Check sheet for the modelled part. Datum: model origin and axes. Units: mm. Round coordinates to 2 decimals unless told otherwise and drop trailing zeros. Write each loop counter-clockwise with the first axis right and the second up, starting at its lowest first coordinate (ties: lowest second). Pieces come first, ordered by that corner, then holes.
Item 1: Section check C-C, the plane y = -19.75. Record the cut outline in (x, z).
Item 2: Section check A-A, the plane z = -7. Record the cut outline in (x, y).
Item 3: Depth check by flat-ended pin: pin 1 (6.5 mm diameter, centred on y = -34.75, z = 83, fed in from -X); pin 2 (3 mm diameter, centred on x = 18.5, z = 81, fed in from +Y); pin 3 (3.5 mm diameter, centred on y = -34.75, z = 53, fed in from -X). Enter the tip coordinate at first touch or a pass-through.
Item 4: Section check B-B, the plane z = 68. Record the cut outline in (x, y), plus the area to 3 significant figures.
Item 5: Material ranges on line 1 along Y through (x, z) = (17.75, -7); line 2 along Z through (x, y) = (17, -19.75); line 3 along Y through (x, z) = (14.5, 83), recorded low to high.
Item 6: Section check D-D, the plane x = 16. State how many separate pieces and enclosed holes the cut face has, plus the area to 3 significant figures.
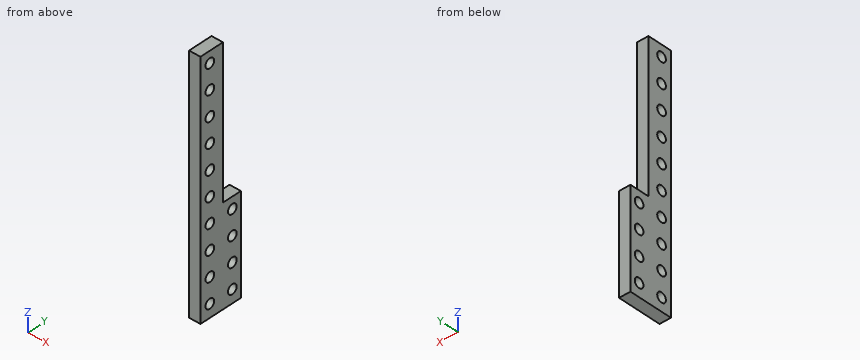
from build123d import *

# Parameters (mm, degrees)
CYLINDER021_R     = 2.9
CYLINDER021_DEPTH = 132
CYLINDER022_R     = 2.9
CYLINDER022_DEPTH = 132
CYLINDER023_R     = 2.9
CYLINDER023_DEPTH = 132
CYLINDER024_R     = 2.9
CYLINDER024_DEPTH = 132
CYLINDER025_R     = 2.9
CYLINDER025_DEPTH = 132
CYLINDER026_R     = 2.9
CYLINDER026_DEPTH = 132
CYLINDER027_R     = 2.9
CYLINDER027_DEPTH = 132
CYLINDER028_R     = 2.9
CYLINDER028_DEPTH = 132
CYLINDER029_R     = 2.9
CYLINDER029_DEPTH = 132
CYLINDER030_R     = 2.9
CYLINDER030_DEPTH = 132
CYLINDER031_R     = 2.9
CYLINDER031_DEPTH = 132
CYLINDER032_R     = 2.9
CYLINDER032_DEPTH = 132
CYLINDER033_R     = 2.9
CYLINDER033_DEPTH = 132
CYLINDER034_R     = 2.9
CYLINDER034_DEPTH = 132
CYLINDER035_R     = 2.9
CYLINDER035_DEPTH = 132
CYLINDER036_R     = 2.9
CYLINDER036_DEPTH = 132
CYLINDER037_R     = 2.9
CYLINDER037_DEPTH = 132
CYLINDER038_R     = 2.9
CYLINDER038_DEPTH = 132
CYLINDER039_R     = 2.9
CYLINDER039_DEPTH = 132
CYLINDER020_R     = 2.9
CYLINDER020_DEPTH = 132
CYLINDER001_R     = 2.9
CYLINDER001_DEPTH = 132
CYLINDER002_R     = 2.9
CYLINDER002_DEPTH = 132
CYLINDER003_R     = 2.9
CYLINDER003_DEPTH = 132
CYLINDER004_R     = 2.9
CYLINDER004_DEPTH = 132
CYLINDER005_R     = 2.9
CYLINDER005_DEPTH = 132
CYLINDER006_R     = 2.9
CYLINDER006_DEPTH = 132
CYLINDER007_R     = 2.9
CYLINDER007_DEPTH = 132
CYLINDER008_R     = 2.9
CYLINDER008_DEPTH = 132
CYLINDER009_R     = 2.9
CYLINDER009_DEPTH = 132
CYLINDER010_R     = 2.9
CYLINDER010_DEPTH = 132
CYLINDER011_R     = 2.9
CYLINDER011_DEPTH = 132
CYLINDER012_R     = 2.9
CYLINDER012_DEPTH = 132
CYLINDER013_R     = 2.9
CYLINDER013_DEPTH = 132
CYLINDER014_R     = 2.9
CYLINDER014_DEPTH = 132
CYLINDER015_R     = 2.9
CYLINDER015_DEPTH = 132
CYLINDER016_R     = 2.9
CYLINDER016_DEPTH = 132
CYLINDER017_R     = 2.9
CYLINDER017_DEPTH = 132
CYLINDER018_R     = 2.9
CYLINDER018_DEPTH = 132
CYLINDER019_R     = 2.9
CYLINDER019_DEPTH = 132
CYLINDER_R        = 2.9
CYLINDER_DEPTH    = 132
CUBE001_W         = 7
CUBE001_H         = 15
CUBE001_DEPTH     = 150
CUBE_W            = 7
CUBE_H            = 12
CUBE_DEPTH        = 60


with BuildPart() as cylinder021:
    # cylinder021 → cylinder021 (new body)
    with BuildSketch(Plane(origin=(-66, 0, 25), x_dir=(0, 0, -1), z_dir=(1, 0, 0))):
        Circle(CYLINDER021_R)
    extrude(amount=CYLINDER021_DEPTH)


with BuildPart() as cylinder022:
    # cylinder022 → cylinder022 (new body)
    with BuildSketch(Plane(origin=(-66, 0, 40), x_dir=(0, 0, -1), z_dir=(1, 0, 0))):
        Circle(CYLINDER022_R)
    extrude(amount=CYLINDER022_DEPTH)


with BuildPart() as cylinder023:
    # cylinder023 → cylinder023 (new body)
    with BuildSketch(Plane(origin=(-66, 0, 55), x_dir=(0, 0, -1), z_dir=(1, 0, 0))):
        Circle(CYLINDER023_R)
    extrude(amount=CYLINDER023_DEPTH)


with BuildPart() as cylinder024:
    # cylinder024 → cylinder024 (new body)
    with BuildSketch(Plane(origin=(-66, 0, 70), x_dir=(0, 0, -1), z_dir=(1, 0, 0))):
        Circle(CYLINDER024_R)
    extrude(amount=CYLINDER024_DEPTH)


with BuildPart() as cylinder025:
    # cylinder025 → cylinder025 (new body)
    with BuildSketch(Plane(origin=(-66, 0, 85), x_dir=(0, 0, -1), z_dir=(1, 0, 0))):
        Circle(CYLINDER025_R)
    extrude(amount=CYLINDER025_DEPTH)


with BuildPart() as cylinder026:
    # cylinder026 → cylinder026 (new body)
    with BuildSketch(Plane(origin=(-66, 0, 100), x_dir=(0, 0, -1), z_dir=(1, 0, 0))):
        Circle(CYLINDER026_R)
    extrude(amount=CYLINDER026_DEPTH)


with BuildPart() as cylinder027:
    # cylinder027 → cylinder027 (new body)
    with BuildSketch(Plane(origin=(-66, 0, 115), x_dir=(0, 0, -1), z_dir=(1, 0, 0))):
        Circle(CYLINDER027_R)
    extrude(amount=CYLINDER027_DEPTH)


with BuildPart() as cylinder028:
    # cylinder028 → cylinder028 (new body)
    with BuildSketch(Plane(origin=(-66, 0, 130), x_dir=(0, 0, -1), z_dir=(1, 0, 0))):
        Circle(CYLINDER028_R)
    extrude(amount=CYLINDER028_DEPTH)


with BuildPart() as cylinder029:
    # cylinder029 → cylinder029 (new body)
    with BuildSketch(Plane(origin=(-66, 0, 145), x_dir=(0, 0, -1), z_dir=(1, 0, 0))):
        Circle(CYLINDER029_R)
    extrude(amount=CYLINDER029_DEPTH)


with BuildPart() as cylinder030:
    # cylinder030 → cylinder030 (new body)
    with BuildSketch(Plane(origin=(-66, 0, 160), x_dir=(0, 0, -1), z_dir=(1, 0, 0))):
        Circle(CYLINDER030_R)
    extrude(amount=CYLINDER030_DEPTH)


with BuildPart() as cylinder031:
    # cylinder031 → cylinder031 (new body)
    with BuildSketch(Plane(origin=(-66, 0, 175), x_dir=(0, 0, -1), z_dir=(1, 0, 0))):
        Circle(CYLINDER031_R)
    extrude(amount=CYLINDER031_DEPTH)


with BuildPart() as cylinder032:
    # cylinder032 → cylinder032 (new body)
    with BuildSketch(Plane(origin=(-66, 0, 190), x_dir=(0, 0, -1), z_dir=(1, 0, 0))):
        Circle(CYLINDER032_R)
    extrude(amount=CYLINDER032_DEPTH)


with BuildPart() as cylinder033:
    # cylinder033 → cylinder033 (new body)
    with BuildSketch(Plane(origin=(-66, 0, 205), x_dir=(0, 0, -1), z_dir=(1, 0, 0))):
        Circle(CYLINDER033_R)
    extrude(amount=CYLINDER033_DEPTH)


with BuildPart() as cylinder034:
    # cylinder034 → cylinder034 (new body)
    with BuildSketch(Plane(origin=(-66, 0, 220), x_dir=(0, 0, -1), z_dir=(1, 0, 0))):
        Circle(CYLINDER034_R)
    extrude(amount=CYLINDER034_DEPTH)


with BuildPart() as cylinder035:
    # cylinder035 → cylinder035 (new body)
    with BuildSketch(Plane(origin=(-66, 0, 235), x_dir=(0, 0, -1), z_dir=(1, 0, 0))):
        Circle(CYLINDER035_R)
    extrude(amount=CYLINDER035_DEPTH)


with BuildPart() as cylinder036:
    # cylinder036 → cylinder036 (new body)
    with BuildSketch(Plane(origin=(-66, 0, 250), x_dir=(0, 0, -1), z_dir=(1, 0, 0))):
        Circle(CYLINDER036_R)
    extrude(amount=CYLINDER036_DEPTH)


with BuildPart() as cylinder037:
    # cylinder037 → cylinder037 (new body)
    with BuildSketch(Plane(origin=(-66, 0, 265), x_dir=(0, 0, -1), z_dir=(1, 0, 0))):
        Circle(CYLINDER037_R)
    extrude(amount=CYLINDER037_DEPTH)


with BuildPart() as cylinder038:
    # cylinder038 → cylinder038 (new body)
    with BuildSketch(Plane(origin=(-66, 0, 280), x_dir=(0, 0, -1), z_dir=(1, 0, 0))):
        Circle(CYLINDER038_R)
    extrude(amount=CYLINDER038_DEPTH)


with BuildPart() as cylinder039:
    # cylinder039 → cylinder039 (new body)
    with BuildSketch(Plane(origin=(-66, 0, 295), x_dir=(0, 0, -1), z_dir=(1, 0, 0))):
        Circle(CYLINDER039_R)
    extrude(amount=CYLINDER039_DEPTH)


with BuildPart() as group001:
    # cylinder020 → cylinder020 (new body)
    with BuildSketch(Plane(origin=(-66, 0, 10), x_dir=(0, 0, -1), z_dir=(1, 0, 0))):
        Circle(CYLINDER020_R)
    extrude(amount=CYLINDER020_DEPTH)

    # Group001: union cylinder021, cylinder022, cylinder023, cylinder024, cylinder025, cylinder026, cylinder027, cylinder028, cylinder029, cylinder030, cylinder031, cylinder032, cylinder033, cylinder034, cylinder035, cylinder036, cylinder037, cylinder038, cylinder039
    add(cylinder021.part)
    add(cylinder022.part)
    add(cylinder023.part)
    add(cylinder024.part)
    add(cylinder025.part)
    add(cylinder026.part)
    add(cylinder027.part)
    add(cylinder028.part)
    add(cylinder029.part)
    add(cylinder030.part)
    add(cylinder031.part)
    add(cylinder032.part)
    add(cylinder033.part)
    add(cylinder034.part)
    add(cylinder035.part)
    add(cylinder036.part)
    add(cylinder037.part)
    add(cylinder038.part)
    add(cylinder039.part)


with BuildPart() as group001_1:
    # Group001 placement: moved
    add(group001.part.moved(Location((0, -34.75, -32))))


with BuildPart() as cylinder001:
    # cylinder001 → cylinder001 (new body)
    with BuildSketch(Plane(origin=(-66, 0, 25), x_dir=(0, 0, -1), z_dir=(1, 0, 0))):
        Circle(CYLINDER001_R)
    extrude(amount=CYLINDER001_DEPTH)


with BuildPart() as cylinder002:
    # cylinder002 → cylinder002 (new body)
    with BuildSketch(Plane(origin=(-66, 0, 40), x_dir=(0, 0, -1), z_dir=(1, 0, 0))):
        Circle(CYLINDER002_R)
    extrude(amount=CYLINDER002_DEPTH)


with BuildPart() as cylinder003:
    # cylinder003 → cylinder003 (new body)
    with BuildSketch(Plane(origin=(-66, 0, 55), x_dir=(0, 0, -1), z_dir=(1, 0, 0))):
        Circle(CYLINDER003_R)
    extrude(amount=CYLINDER003_DEPTH)


with BuildPart() as cylinder004:
    # cylinder004 → cylinder004 (new body)
    with BuildSketch(Plane(origin=(-66, 0, 70), x_dir=(0, 0, -1), z_dir=(1, 0, 0))):
        Circle(CYLINDER004_R)
    extrude(amount=CYLINDER004_DEPTH)


with BuildPart() as cylinder005:
    # cylinder005 → cylinder005 (new body)
    with BuildSketch(Plane(origin=(-66, 0, 85), x_dir=(0, 0, -1), z_dir=(1, 0, 0))):
        Circle(CYLINDER005_R)
    extrude(amount=CYLINDER005_DEPTH)


with BuildPart() as cylinder006:
    # cylinder006 → cylinder006 (new body)
    with BuildSketch(Plane(origin=(-66, 0, 100), x_dir=(0, 0, -1), z_dir=(1, 0, 0))):
        Circle(CYLINDER006_R)
    extrude(amount=CYLINDER006_DEPTH)


with BuildPart() as cylinder007:
    # cylinder007 → cylinder007 (new body)
    with BuildSketch(Plane(origin=(-66, 0, 115), x_dir=(0, 0, -1), z_dir=(1, 0, 0))):
        Circle(CYLINDER007_R)
    extrude(amount=CYLINDER007_DEPTH)


with BuildPart() as cylinder008:
    # cylinder008 → cylinder008 (new body)
    with BuildSketch(Plane(origin=(-66, 0, 130), x_dir=(0, 0, -1), z_dir=(1, 0, 0))):
        Circle(CYLINDER008_R)
    extrude(amount=CYLINDER008_DEPTH)


with BuildPart() as cylinder009:
    # cylinder009 → cylinder009 (new body)
    with BuildSketch(Plane(origin=(-66, 0, 145), x_dir=(0, 0, -1), z_dir=(1, 0, 0))):
        Circle(CYLINDER009_R)
    extrude(amount=CYLINDER009_DEPTH)


with BuildPart() as cylinder010:
    # cylinder010 → cylinder010 (new body)
    with BuildSketch(Plane(origin=(-66, 0, 160), x_dir=(0, 0, -1), z_dir=(1, 0, 0))):
        Circle(CYLINDER010_R)
    extrude(amount=CYLINDER010_DEPTH)


with BuildPart() as cylinder011:
    # cylinder011 → cylinder011 (new body)
    with BuildSketch(Plane(origin=(-66, 0, 175), x_dir=(0, 0, -1), z_dir=(1, 0, 0))):
        Circle(CYLINDER011_R)
    extrude(amount=CYLINDER011_DEPTH)


with BuildPart() as cylinder012:
    # cylinder012 → cylinder012 (new body)
    with BuildSketch(Plane(origin=(-66, 0, 190), x_dir=(0, 0, -1), z_dir=(1, 0, 0))):
        Circle(CYLINDER012_R)
    extrude(amount=CYLINDER012_DEPTH)


with BuildPart() as cylinder013:
    # cylinder013 → cylinder013 (new body)
    with BuildSketch(Plane(origin=(-66, 0, 205), x_dir=(0, 0, -1), z_dir=(1, 0, 0))):
        Circle(CYLINDER013_R)
    extrude(amount=CYLINDER013_DEPTH)


with BuildPart() as cylinder014:
    # cylinder014 → cylinder014 (new body)
    with BuildSketch(Plane(origin=(-66, 0, 220), x_dir=(0, 0, -1), z_dir=(1, 0, 0))):
        Circle(CYLINDER014_R)
    extrude(amount=CYLINDER014_DEPTH)


with BuildPart() as cylinder015:
    # cylinder015 → cylinder015 (new body)
    with BuildSketch(Plane(origin=(-66, 0, 235), x_dir=(0, 0, -1), z_dir=(1, 0, 0))):
        Circle(CYLINDER015_R)
    extrude(amount=CYLINDER015_DEPTH)


with BuildPart() as cylinder016:
    # cylinder016 → cylinder016 (new body)
    with BuildSketch(Plane(origin=(-66, 0, 250), x_dir=(0, 0, -1), z_dir=(1, 0, 0))):
        Circle(CYLINDER016_R)
    extrude(amount=CYLINDER016_DEPTH)


with BuildPart() as cylinder017:
    # cylinder017 → cylinder017 (new body)
    with BuildSketch(Plane(origin=(-66, 0, 265), x_dir=(0, 0, -1), z_dir=(1, 0, 0))):
        Circle(CYLINDER017_R)
    extrude(amount=CYLINDER017_DEPTH)


with BuildPart() as cylinder018:
    # cylinder018 → cylinder018 (new body)
    with BuildSketch(Plane(origin=(-66, 0, 280), x_dir=(0, 0, -1), z_dir=(1, 0, 0))):
        Circle(CYLINDER018_R)
    extrude(amount=CYLINDER018_DEPTH)


with BuildPart() as cylinder019:
    # cylinder019 → cylinder019 (new body)
    with BuildSketch(Plane(origin=(-66, 0, 295), x_dir=(0, 0, -1), z_dir=(1, 0, 0))):
        Circle(CYLINDER019_R)
    extrude(amount=CYLINDER019_DEPTH)


with BuildPart() as union:
    # cylinder → cylinder (new body)
    with BuildSketch(Plane(origin=(-66, 0, 10), x_dir=(0, 0, -1), z_dir=(1, 0, 0))):
        Circle(CYLINDER_R)
    extrude(amount=CYLINDER_DEPTH)

    # Group: union cylinder001, cylinder002, cylinder003, cylinder004, cylinder005, cylinder006, cylinder007, cylinder008, cylinder009, cylinder010, cylinder011, cylinder012, cylinder013, cylinder014, cylinder015, cylinder016, cylinder017, cylinder018, cylinder019
    add(cylinder001.part)
    add(cylinder002.part)
    add(cylinder003.part)
    add(cylinder004.part)
    add(cylinder005.part)
    add(cylinder006.part)
    add(cylinder007.part)
    add(cylinder008.part)
    add(cylinder009.part)
    add(cylinder010.part)
    add(cylinder011.part)
    add(cylinder012.part)
    add(cylinder013.part)
    add(cylinder014.part)
    add(cylinder015.part)
    add(cylinder016.part)
    add(cylinder017.part)
    add(cylinder018.part)
    add(cylinder019.part)


with BuildPart() as union_1:
    # Group placement: moved
    add(union.part.moved(Location((0, -19.75, -32))))

    # union: union Group001
    add(group001_1.part)


with BuildPart() as cube001:
    # cube001 → cube001 (new body)
    with BuildSketch(Plane(origin=(-3.5, -21, -30), x_dir=(1, 0, 0), z_dir=(0, 0, 1))):
        with Locations((3.5, 7.5)):
            Rectangle(CUBE001_W, CUBE001_H)
    extrude(amount=CUBE001_DEPTH)


with BuildPart() as difference:
    # cube → cube (new body)
    with BuildSketch(Plane(origin=(-3.5, -6, -30), x_dir=(1, 0, 0), z_dir=(0, 0, 1))):
        with Locations((3.5, 6)):
            Rectangle(CUBE_W, CUBE_H)
    extrude(amount=CUBE_DEPTH)

    # Matrix_Union: union cube001
    add(cube001.part)


with BuildPart() as difference_1:
    # Matrix_Union placement: moved
    add(difference.part.moved(Location((16.5, -20, 0))))

    # difference: cut union
    add(union_1.part, mode=Mode.SUBTRACT)


solid = difference_1.part
Values found:
1. outline: (13, -30) - (20, -30) - (20, -24.9) - (13, -24.9) - close; (13, -19.1) - (20, -19.1) - (20, -9.9) - (13, -9.9) - close; (13, -4.1) - (20, -4.1) - (20, 5.1) - (13, 5.1) - close; (13, 10.9) - (20, 10.9) - (20, 20.1) - (13, 20.1) - close; (13, 25.9) - (20, 25.9) - (20, 30) - (13, 30) - close
2. outline: (13, -41) - (20, -41) - (20, -37.65) - (13, -37.65) - close; (13, -31.85) - (20, -31.85) - (20, -22.65) - (13, -22.65) - close; (13, -16.85) - (20, -16.85) - (20, -14) - (13, -14) - close
3. pin 1: stops at x = 13
3. pin 2: stops at y = -26
3. pin 3: passes through
4. outline: (13, -41) - (20, -41) - (20, -37.65) - (13, -37.65) - close; (13, -31.85) - (20, -31.85) - (20, -26) - (13, -26) - close
4. area: 64.4 mm2
5. line 1: y = -41 to -37.65, -31.85 to -22.65, -16.85 to -14
5. line 2: z = -30 to -24.9, -19.1 to -9.9, -4.1 to 5.1, 10.9 to 20.1, 25.9 to 30
5. line 3: y = -41 to -37.65, -31.85 to -26
6. separate pieces: 1
6. enclosed holes: 14
6. area: 2,600 mm2
